```python
from build123d import *

# Parameters (mm, degrees)
SKETCH1_W           = 89
SKETCH1_H           = 51
SKETCH1_R           = 2.5
BOSS_EXTRUDE1_DEPTH = 3
SKETCH2_R           = 5.5
SKETCH2_R_2         = 2.5
BOSS_EXTRUDE2_DEPTH = 3
SKETCH3_W           = 93
SKETCH3_H           = 55
SKETCH3_W_2         = 89
SKETCH3_H_2         = 51
BOSS_EXTRUDE3_DEPTH = 20
CHAMFER1_SIZE       = 2
CHAMFER2_SIZE       = 1


with BuildPart() as part:
    # Sketch1 → Boss-Extrude1 (new body)
    with BuildSketch(Plane(origin=(0, 0, 0), x_dir=(1, 0, 0), z_dir=(0, 1, 0))):
        with Locations((36.5, -17.5)):
            Rectangle(SKETCH1_W, SKETCH1_H)
        with Locations(Location((0, 0, 0), (0, 0, 270))):
            Circle(SKETCH1_R, mode=Mode.SUBTRACT)
        with Locations(Location((73, 0, 0), (0, 0, 270))):
            Circle(SKETCH1_R, mode=Mode.SUBTRACT)
        with Locations(Location((0, -35, 0), (0, 0, 270))):
            Circle(SKETCH1_R, mode=Mode.SUBTRACT)
        with Locations(Location((73, -35, 0), (0, 0, 270))):
            Circle(SKETCH1_R, mode=Mode.SUBTRACT)
    extrude(amount=BOSS_EXTRUDE1_DEPTH)

    # Sketch2 → Boss-Extrude2 (add)
    # profile 1 of 4: a face of its own
    with BuildSketch(Plane(origin=(0, 3, 0), x_dir=(1, 0, 0), z_dir=(0, 1, 0))):
        with Locations(Location((0, 0, 0), (0, 0, 270))):
            Circle(SKETCH2_R)
        with Locations(Location((0, 0, 0), (0, 0, 270))):
            Circle(SKETCH2_R_2, mode=Mode.SUBTRACT)
    # profile 2 of 4: a face of its own
    with BuildSketch(Plane(origin=(0, 3, 0), x_dir=(1, 0, 0), z_dir=(0, 1, 0))):
        with Locations(Location((73, 0, 0), (0, 0, 270))):
            Circle(SKETCH2_R)
        with Locations(Location((73, 0, 0), (0, 0, 270))):
            Circle(SKETCH2_R_2, mode=Mode.SUBTRACT)
    # profile 3 of 4: a face of its own
    with BuildSketch(Plane(origin=(0, 3, 0), x_dir=(1, 0, 0), z_dir=(0, 1, 0))):
        with Locations(Location((73, -35, 0), (0, 0, 270))):
            Circle(SKETCH2_R)
        with Locations(Location((73, -35, 0), (0, 0, 270))):
            Circle(SKETCH2_R_2, mode=Mode.SUBTRACT)
    # profile 4 of 4: a face of its own
    with BuildSketch(Plane(origin=(0, 3, 0), x_dir=(1, 0, 0), z_dir=(0, 1, 0))):
        with Locations(Location((0, -35, 0), (0, 0, 270))):
            Circle(SKETCH2_R)
        with Locations(Location((0, -35, 0), (0, 0, 270))):
            Circle(SKETCH2_R_2, mode=Mode.SUBTRACT)
    extrude(amount=BOSS_EXTRUDE2_DEPTH)

    # Sketch3 → Boss-Extrude3 (add)
    with BuildSketch(Plane.XZ):
        with Locations((36.5, 17.5)):
            Rectangle(SKETCH3_W, SKETCH3_H)
        with Locations((36.5, 17.5)):
            Rectangle(SKETCH3_W_2, SKETCH3_H_2, mode=Mode.SUBTRACT)
    extrude(amount=-BOSS_EXTRUDE3_DEPTH)

    # Chamfer1
    chamfer1_edges = [part.edges().sort_by_distance(p)[0] for p in [
        (-10, 10, 45),
        (83, 10, 45),
        (83, 10, -10),
        (-10, 10, -10),
    ]]
    chamfer(chamfer1_edges, length=CHAMFER1_SIZE)

    # Chamfer2
    chamfer2_edges = [part.edges().sort_by_distance(p)[0] for p in [
        (81, 11.5, 43),
        (81, 11.5, -8),
        (-8, 11.5, -8),
        (-8, 11.5, 43),
    ]]
    chamfer(chamfer2_edges, length=CHAMFER2_SIZE)


solid = part.part
```
For this review, take the finished solid that the model builds, in its own axes (mm). A direction names the side the tool comes from. Give positions to 0.01 mm unless a question says otherwise; leave off trailing zeros. Write each loop counter-clockwise with the first axis right and the second up, starting at its lowest first coordinate (ties: lowest second). Pieces come first, ordered by that corner, then holes.
Item 1: Take a section at B-B (x = 0). Give the boundary of the cut face in (y, z), and give its area (3 significant figures).
Item 2: The part is to be moulded in two halves that separate along Z. For faces 3 (the face through (70.78, 2.96, 36.15)), 4 (the face through (36, 0, 18)), 5 (the face through (36, 10, 45)), say which applies: +Z half, -Z half, draft (parallel to the pull), parting line (faces both ways), or undercut.
Item 3: Wall thickness on probe 1 along X at (y, z) = (1.35, 35); probe 2 along X at (y, z) = (4.65, 35); probe 3 along X at (y, z) = (11.25, 24.5): over which ranges is each line inside the solid? List them lowest first.
Item 4: Take a section at D-D (x = 17.5). Give the boundary of the cut face in (y, z), and give its area (3 significant figures).
Item 5: Machinability: for faces 1 (the face through (78.453, 4.479, -0.716)), 2 (the face through (83, 10, 17)), which of the approach directions +Z, -Z, +X, -X, +Y, -Y give a long, thin tool a straight path to every point of the face, cutting with its end or side? Answer none if there is none.
Item 6: Take a section at A-A (y = 18.75). Give the boundary of the cut face in (x, z), and give its area (3 significant figures).
Item 7: Take a section at C-C (z = 0). Give the boundary of the cut face in (x, y), and give its area (3 significant figures).
Item 8: Insertion check: P1, Ø12, axis at x = 1, z = -1.5, coming from the +Y side; P2, Ø5, axis at x = 6, z = 28, coming from the -Y side; P3, Ø15.5, axis at x = 28, z = 17, coming from the +Y side. Each pin has a flat end and moves straight along its axis. Give the tip position at first contact, or say it passes through.
Established:
1. outline: (0, -10) - (20, -10) - (20, -8) - (3, -8) - (3, -5.5) - (6, -5.5) - (6, -2.5) - (0, -2.5) - close; (0, 2.5) - (6, 2.5) - (6, 5.5) - (3, 5.5) - (3, 29.5) - (6, 29.5) - (6, 32.5) - (0, 32.5) - close; (0, 37.5) - (6, 37.5) - (6, 40.5) - (3, 40.5) - (3, 43) - (20, 43) - (20, 45) - (0, 45) - close
1. area: 239 mm2
2. face 3: undercut
2. face 4: draft
2. face 5: +Z half
3. probe 1: x = -10 to -2.5, 2.5 to 70.5, 75.5 to 83
3. probe 2: x = -10 to -8, -5.5 to -2.5, 2.5 to 5.5, 67.5 to 70.5, 75.5 to 78.5, 81 to 83
3. probe 3: x = -10 to -8, 81 to 83
4. outline: (0, -10) - (20, -10) - (20, -8) - (3, -8) - (3, 43) - (20, 43) - (20, 45) - (0, 45) - close
4. area: 233 mm2
5. face 1: +Y
5. face 2: +Z, -Z, +X, +Y, -Y
6. outline: (-10, -8) - (-8, -10) - (81, -10) - (83, -8) - (83, 43) - (81, 45) - (-8, 45) - (-10, 43) - close; hole (-8, -7) - (-7, -8) - (80, -8) - (81, -7) - (81, 42) - (80, 43) - (-7, 43) - (-8, 42) - close
6. area: 570 mm2
7. outline: (-10, 0) - (-2.5, 0) - (-2.5, 6) - (-5.5, 6) - (-5.5, 3) - (-8, 3) - (-8, 20) - (-10, 20) - close; (2.5, 0) - (70.5, 0) - (70.5, 6) - (67.5, 6) - (67.5, 3) - (5.5, 3) - (5.5, 6) - (2.5, 6) - close; (75.5, 0) - (83, 0) - (83, 20) - (81, 20) - (81, 3) - (78.5, 3) - (78.5, 6) - (75.5, 6) - close
7. area: 353 mm2
8. P1: stops at y = 6
8. P2: stops at y = 0
8. P3: stops at y = 3
